from build123d import *

# Parameters (mm, degrees)
SKETCH1_R           = 35
SKETCH1_R_2         = 30
SKETCH1_R_3         = 25
BOSS_EXTRUDE1_DEPTH = 4
SKETCH2_R           = 3.9
BOSS_EXTRUDE2_DEPTH = 7.1
SKETCH3_R           = 1.6
CUT_EXTRUDE1_DEPTH  = 15
SKETCH4_R           = 2.7
CUT_EXTRUDE2_DEPTH  = 3.2
BOSS_EXTRUDE3_DEPTH = 4.5
BOSS_EXTRUDE4_DEPTH = 4.5
SKETCH8_R           = 3.9
CUT_EXTRUDE3_DEPTH  = 12.5


with BuildPart() as part:
    # Sketch1 → Boss-Extrude1 (new body)
    with BuildSketch(Plane.XY):
        Circle(SKETCH1_R)
        Circle(SKETCH1_R_2, mode=Mode.SUBTRACT)
        Circle(SKETCH1_R_2)
        Circle(SKETCH1_R_3, mode=Mode.SUBTRACT)
    extrude(amount=BOSS_EXTRUDE1_DEPTH)

    # Sketch2 → Boss-Extrude2 (add)
    with BuildSketch(Plane(origin=(0, 0, 0), x_dir=(-1, 0, 0), z_dir=(0, 0, -1))):
        with Locations((0, 30)):
            Circle(SKETCH2_R)
        with Locations((25.980762114, -15)):
            Circle(SKETCH2_R)
        with Locations((-25.980762114, -15)):
            Circle(SKETCH2_R)
    extrude(amount=BOSS_EXTRUDE2_DEPTH)

    # Sketch3 → Cut-Extrude1 (cut)
    with BuildSketch(Plane(origin=(0, 0, -7.1), x_dir=(-1, 0, 0), z_dir=(0, 0, -1))):
        with Locations((0, 30)):
            Circle(SKETCH3_R)
        with Locations((25.980762114, -15)):
            Circle(SKETCH3_R)
        with Locations((-25.980762114, -15)):
            Circle(SKETCH3_R)
    extrude(amount=-CUT_EXTRUDE1_DEPTH, mode=Mode.SUBTRACT)

    # Sketch4 → Cut-Extrude2 (cut)
    with BuildSketch(Plane.XY.offset(4)):
        with Locations((0, 30)):
            Circle(SKETCH4_R)
        with Locations((25.980762114, -15)):
            Circle(SKETCH4_R)
        with Locations((-25.980762114, -15)):
            Circle(SKETCH4_R)
    extrude(amount=-CUT_EXTRUDE2_DEPTH, mode=Mode.SUBTRACT)

    # Sketch6 → Boss-Extrude3 (add)
    with BuildSketch(Plane.XY.offset(4)):
        with BuildLine():
            Line((25.980762114, 15), (27.712812921, 16))
            ThreePointArc((27.712812921, 16), (22.627416998, 22.627416998), (16, 27.712812921))
            Line((16, 27.712812921), (15, 25.980762114))
            ThreePointArc((15, 25.980762114), (21.213203436, 21.213203436), (25.980762114, 15))
        make_face()
    extrude(amount=BOSS_EXTRUDE3_DEPTH)

    # Sketch7 → Boss-Extrude4 (add)
    with BuildSketch(Plane.XY.offset(4)):
        with BuildLine():
            Line((16, -27.712812921), (15, -25.980762114))
            ThreePointArc((15, -25.980762114), (7.764571353, -28.977774789), (0, -30))
            Line((0, -30), (0, -32))
            ThreePointArc((0, -32), (8.282209443, -30.909626441), (16, -27.712812921))
        make_face()
        with BuildLine():
            Line((25.980762114, 15), (27.712812921, 16))
            ThreePointArc((27.712812921, 16), (22.627416998, 22.627416998), (16, 27.712812921))
            Line((16, 27.712812921), (15, 25.980762114))
            ThreePointArc((15, 25.980762114), (21.213203436, 21.213203436), (25.980762114, 15))
        make_face()
        with BuildLine():
            Line((-32, 0), (-30, 0))
            ThreePointArc((-30, 0), (-28.977774789, 7.764571353), (-25.980762114, 15))
            Line((-25.980762114, 15), (-27.712812921, 16))
            ThreePointArc((-27.712812921, 16), (-30.909626441, 8.282209443), (-32, 0))
        make_face()
    extrude(amount=BOSS_EXTRUDE4_DEPTH)

    # Sketch8 → Cut-Extrude3 (cut)
    with BuildSketch(Plane(origin=(0, 0, 0), x_dir=(-1, 0, 0), z_dir=(0, 0, -1))):
        with Locations((0, 30)):
            Circle(SKETCH8_R)
        with Locations((25.980762114, -15)):
            Circle(SKETCH8_R)
        with Locations((-25.980762114, -15)):
            Circle(SKETCH8_R)
    extrude(amount=CUT_EXTRUDE3_DEPTH, mode=Mode.SUBTRACT)


solid = part.part
Design review of the part built by this model. Coordinates are the model's own, in mm. A direction names the side the tool comes from. Round coordinates to 2 decimals unless told otherwise and drop trailing zeros. Write each loop counter-clockwise with the first axis right and the second up, starting at its lowest first coordinate (ties: lowest second). Pieces come first, ordered by that corner, then holes. Notation, with made-up numbers: (54, -21) - (104, -21) arc R18 cw to (104, -1) - close; hole circle Ø8 at (-30, -37.75). An arc over 180 degrees is marked (long way). Use a Markdown table: item, result. Add a question column.
1. For faces 1 (the face through (-29.006, 7.658, 6.219)), 2 (the face through (-26.332, -12.323, 2.422)), 3 (the face through (-31, 0, 6)), list the 3-axis set-ups (+Z, -Z, +X, -X, +Y, -Y) from which the entire face can be reached by the end or side of a thin tool; tool diameter is ignored.
2. Mouldability with a two-part tool opening along X and no side actions: class faces 4 (the face through (-30, 8, 8.5)), 5 (the face through (7.87, -28.95, 6.22)), 6 (the face through (25.629, -12.323, 2.422)) as +X half, -X half, draft (parallel to the pull), parting line (faces both ways), or undercut.
3. We need section C-C (y = -23). State the section outline as (x, z) points.
4. We need section D-D (x = 18.5). State the section outline as (y, z) points.
5. Wall thickness on probe 1 along Y at (x, z) = (0, 0.3); probe 2 along Y at (x, z) = (0, 1.8); probe 3 along Y at (x, z) = (0.5, 4.25): over which ranges is each line inside the solid? List them lowest first.
6. We need section A-A (z = 5). State the section outline as (x, y) points, then the cut area to 3 significant figures.
7. We need section B-B (x = -19). State the section outline as (y, z) points.
8. Clearance check with flat-ended pins moving along their axes: pin 1 (1.5 mm diameter, centred on x = -13, z = 6.5, fed in from -Y); pin 2 (0.6 mm diameter, centred on x = -31, z = 6.5, fed in from -Y); pin 3 (5 mm diameter, centred on y = 16, z = 4, fed in from -X); pin 4 (6 mm diameter, centred on x = 26.5, y = -15, fed in from +Z). State where each tip first meets the part, or that it passes through.
Output:
| question | item | result |
|---|---|---|
| 1 | face 1 | +Z, +X, -Y |
| 1 | face 2 | +Z |
| 1 | face 3 | +Z, +X, -X, -Y |
| 2 | face 4 | draft |
| 2 | face 5 | -X half |
| 2 | face 6 | undercut |
| 3 | outline | (-26.38, 0) - (-9.8, 0) - (-9.8, 4) - (-26.38, 4) - close; (9.8, 0) - (26.38, 0) - (26.38, 4) - (9.8, 4) - close |
| 4 | outline | (-29.71, 0) - (-16.82, 0) - (-16.82, 4) - (-29.71, 4) - close; (16.82, 0) - (29.71, 0) - (29.71, 4) - (26.11, 4) - (26.11, 8.5) - (23.62, 8.5) - (23.62, 4) - (16.82, 4) - close |
| 5 | probe 1 | y = -35 to -25, 25 to 28.4, 31.6 to 35 |
| 5 | probe 2 | y = -35 to -25, 25 to 27.3, 32.7 to 35 |
| 5 | probe 3 | y = -32 to -30 |
| 6 | outline | (-32, 0) - (-30, 0) arc R30 cw to (-25.98, 15) - (-27.71, 16) arc R32 ccw to start; (0, -32) arc R32 ccw to (16, -27.71) - (15, -25.98) arc R30 cw to (0, -30) - close; (15, 25.98) arc R30 cw to (25.98, 15) - (27.71, 16) arc R32 ccw to (16, 27.71) - close |
| 6 | area | 97.4 mm2 |
| 7 | outline | (-29.39, 0) - (-16.25, 0) - (-16.25, 4) - (-29.39, 4) - close; (16.25, 0) - (29.39, 0) - (29.39, 4) - (16.25, 4) - close |
| 8 | pin 1 | passes through |
| 8 | pin 2 | stops at y = 0 |
| 8 | pin 3 | stops at x = -32.29 |
| 8 | pin 4 | stops at z = 4 |
